Work out the finished part from the listing and answer in its coordinate system (mm). A direction names the side the tool comes from. Give positions to 0.01 mm unless a question says otherwise; leave off trailing zeros. Order: outer loops, then holes, each group sorted by start corner. A loop starts at its lowest first (then second) coordinate and runs counter-clockwise, first axis right, second up.
```python
from build123d import *

# Parameters (mm, degrees)
F3_R     = 5
F5_D     = 15
F5_DEPTH = 28.576000561


# Not quite as in the source:
# - a fillet or chamfer that OpenCascade refuses, or shapes differently, is made with other operations: its cross-section is extruded or revolved along the edge and cut away or added


with BuildPart() as f1:
    # F0 (on Front) → F1 (revolve)
    with BuildSketch(Plane.XZ):
        Polygon((26.3250011413, 145), (-27.2249993616, 145), (-28.575000561, 145), (-28.575000561, 100), (0, 100), (8.3250019151, 114.3999986072), (26.3250011413, 114.3999986072), align=None)
    revolve(axis=Axis((-1.3500031339, 0, 0), (1, 0, 0)))

    # F2: chamfer of 5 on 4 edges, made by hand

    # F2_s1 → F2_t2 (revolve, cut)
    with BuildSketch(Plane.XZ):
        Polygon((26.3250011413, 140), (21.3250011413, 145), (26.3250011413, 145), align=None)
    revolve(axis=Axis((26.3250011413, 0, 0), (1, 0, 0)), mode=Mode.SUBTRACT)

    # F2_s3 → F2_t4 (revolve, cut)
    with BuildSketch(Plane.XZ):
        Polygon((21.3250011413, 114.3999986072), (26.3250011413, 119.3999986072), (26.3250011413, 114.3999986072), align=None)
    revolve(axis=Axis((26.3250011413, 0, 0), (1, 0, 0)), mode=Mode.SUBTRACT)

    # F2_s5 → F2_t6 (revolve, cut)
    with BuildSketch(Plane.XZ):
        Polygon((-2.8848150214, 100), (1.4438587798, 102.4974846409), (0, 100), align=None)
    revolve(axis=Axis((0, 0, 0), (1, 0, 0)), mode=Mode.SUBTRACT)

    # F2_s7 → F2_t8 (revolve, cut)
    with BuildSketch(Plane.XZ):
        Polygon((-23.575000561, 145), (-28.575000561, 140), (-28.575000561, 145), align=None)
    revolve(axis=Axis((-28.575000561, 0, 0), (1, 0, 0)), mode=Mode.SUBTRACT)

    # F3
    f3_edges = [f1.edges().sort_by_distance(p)[0] for p in [
        (8.325002, 0, -114.399999),
    ]]
    fillet(f3_edges, radius=F3_R)

    # F5 (through all, one way)
    with BuildSketch(Plane.YZ):
        with Locations((0, 130.4700821638)):
            Circle(F5_D / 2)
    extrude(amount=-F5_DEPTH, mode=Mode.SUBTRACT)


solid = f1.part
```
1. Straight lines are drawn through the part: probe 1 along Z at (x, y) = (-15, 0); probe 2 along Z at (x, y) = (13.75, 0); probe 3 along Y at (x, z) = (-20.25, 0). For each, find the intervals that lie inside material, in ascending order.
Findings below:
probe 1: z = -145 to -100, 100 to 122.97, 137.97 to 145
probe 2: z = -145 to -114.4, 114.4 to 145
probe 3: y = -145 to -100, 100 to 145
2. The part is cut by section A-A (x = 15). Write down the section's boundary in (y, z).
Findings below:
outline: circle Ø290 at (0, 0); hole circle Ø228.8 at (0, 0)
3. The part is cut by section B-B (x = -8). Write down the section's boundary in (y, z), then the cut area to 3 significant figures.
Findings below:
outline: circle Ø290 at (0, 0); hole circle Ø200 at (0, 0); hole circle Ø15 at (0, 130.47)
area: 34,500 mm2
4. Which of the six approach directions +Z, -Z, +X, -X, +Y, -Y give full straight-line access (tool end or side, diameter ignored) to faces 1 (the face through (26.325, -63, -103)), 2 (the face through (-14.087, -0.976, 137.906)), 3 (the face through (16.338, -113.426, -14.893))?
Findings below:
face 1: +Z, -Z, +X, +Y, -Y
face 2: -X
face 3: +X
5. The mould has two halves that part along Y. Classify faces 4 (the face through (-1.439, -43.554, 138.304)), 5 (the face through (-15.55, -30.04, 95.38)), 6 (the face through (-28.575, -33, -95)): pulls with the +Y half, pulls with the -Y half, needs draft (parallel to the pull), parting line crosses it, or undercut.
Findings below:
face 4: parting line crosses it
face 5: undercut
face 6: needs draft
6. Given P1, Ø2, axis at x = 18, z = 23, coming from the -Y side; P2, Ø8, axis at x = 9.5, z = 103, coming from the +Y side; P3, Ø8, axis at x = 3, y = -23, coming from the -Z side, each flat-ended and moving along its own axis, determine where each tip first touches the part or whether it passes through.
Findings below:
P1: stops at y = -143.32
P2: stops at y = 105.94
P3: stops at z = -143.75
